The listing builds one solid part. Answer for the finished solid, in the listing's coordinates (mm). A direction names the side the tool comes from. Coordinates: 2 decimals unless noted, no trailing zeros. Write each loop counter-clockwise with the first axis right and the second up, starting at its lowest first coordinate (ties: lowest second). Pieces come first, ordered by that corner, then holes.
(1) Straight lines are drawn through the part: line 1 (Y direction, x = -12.5, z = 2.5); line 2 (X direction, y = 163, z = 4); line 3 (Y direction, x = -48.5, z = -1.5). For each, find the intervals that lie inside material, in ascending order.
(2) For a pull along Y with two mould halves and no side action, classify faces 6 (the flat face through (68, 129, 4.762)), 7 (the flat face through (-24, 197, 0)), 8 (the flat face through (-80, 197, 4.762)) as +Y half, -Y half, draft (parallel to the pull), parting line (faces both ways), or undercut.
(3) Which of the six approach directions +Z, -Z, +X, -X, +Y, -Y give full straight-line access (tool end or side, diameter ignored) to faces 1 (the flat face through (0, 118, 4.762)), 2 (the flat face through (68, 265, 4.762)), 3 (the flat face through (-69, 129, 4.762)), 4 (the flat face through (0, 276, 4.762)), 5 (the flat face through (-69, 265, 4.762))?
(4) The part is cut by section B-B on y = 95. Determine the outline of the cut face in (x, z).
(5) The part is cut by section A-A on x = 135.5. Determine the outline of the cut face in (y, z).
(6) The part is cut by section D-D on x = -44. Give the number of separate pieces and of enclosed holes in the cut face, plus the area to 3 significant figures.
(7) The part is cut by section C-C on z = -1.5. Determine the outline of the cut face in (x, y).
(8) Given P1, Ø9.5, axis at x = -86.5, y = 189, coming from the +Z side; P2, Ø3, axis at y = 130, z = 1, coming from the -X side; P3, Ø3, axis at x = -133.5, y = 176, coming from the -Z side; P4, Ø8, axis at x = 139.5, y = 163.5, coming from the +Z side, each flat-ended and moving along its own axis, determine where each tip first touches the part or whether it passes through.
from build123d import *
from OCP.BRepFilletAPI import BRepFilletAPI_MakeChamfer

# Parameters (mm, degrees)
SKETCH1_W           = 31.75
SKETCH1_H           = 38.1
SKETCH1_H_2         = 6.35
SKETCH1_W_2         = 6.35
SKETCH1_H_3         = 31.75
SKETCH1_W_3         = 38.1
BOSS_EXTRUDE1_DEPTH = 4.7625
SKETCH1_4_W         = 6.35
SKETCH1_4_H         = 31.75
SKETCH1_4_W_2       = 38.1
SKETCH1_4_W_3       = 31.75
SKETCH1_4_H_2       = 6.35
SKETCH1_4_H_3       = 38.1
BOSS_EXTRUDE2_DEPTH = 3.175
SKETCH1_5_W         = 38.1
SKETCH1_5_H         = 6.35
SKETCH1_5_W_2       = 63.5
SKETCH1_5_W_3       = 6.35
SKETCH1_5_H_2       = 38.1
SKETCH1_5_W_4       = 19.05
SKETCH1_5_H_3       = 139.7
SKETCH1_5_H_4       = 19.05
SKETCH1_5_H_5       = 158.75
SKETCH1_5_H_6       = 31.75
SKETCH1_5_W_5       = 31.75
BOSS_EXTRUDE3_DEPTH = 6.35
CHAMFER1_SIZE       = 25.4
CHAMFER1_SIZE2      = 3.175
CHAMFER2_SIZE       = 3.175
CHAMFER2_SIZE2      = 25.4
CHAMFER3_SIZE       = 38.1
CHAMFER3_SIZE2      = 3.175


with BuildPart() as part:
    # Sketch1 → Boss-Extrude1 (new body)
    with BuildSketch(Plane.XY):
        Polygon((-63.5, 171.45), (-95.25, 171.45), (-95.25, 101.6), (-25.4, 101.6), (-25.4, 133.35), (-63.5, 133.35), align=None)
        with Locations((-79.375, 196.85)):
            Rectangle(SKETCH1_W, SKETCH1_H)
        with Locations((-79.375, 174.625)):
            Rectangle(SKETCH1_W, SKETCH1_H_2)
        with Locations((-79.375, 219.075)):
            Rectangle(SKETCH1_W, SKETCH1_H_2)
        Polygon((-25.4, 260.35), (-25.4, 292.1), (-95.25, 292.1), (-95.25, 222.25), (-63.5, 222.25), (-63.5, 260.35), align=None)
        with Locations((-22.225, 276.225)):
            Rectangle(SKETCH1_W_2, SKETCH1_H_3)
        with Locations((0, 276.225)):
            Rectangle(SKETCH1_W_3, SKETCH1_H_3)
        with Locations((22.225, 276.225)):
            Rectangle(SKETCH1_W_2, SKETCH1_H_3)
        Polygon((95.25, 292.1), (25.4, 292.1), (25.4, 260.35), (63.5, 260.35), (63.5, 222.25), (95.25, 222.25), align=None)
        with Locations((79.375, 219.075)):
            Rectangle(SKETCH1_W, SKETCH1_H_2)
        with Locations((79.375, 196.85)):
            Rectangle(SKETCH1_W, SKETCH1_H)
        with Locations((79.375, 174.625)):
            Rectangle(SKETCH1_W, SKETCH1_H_2)
        Polygon((95.25, 101.6), (95.25, 171.45), (63.5, 171.45), (63.5, 133.35), (25.4, 133.35), (25.4, 101.6), align=None)
        with Locations((22.225, 117.475)):
            Rectangle(SKETCH1_W_2, SKETCH1_H_3)
        with Locations((0, 117.475)):
            Rectangle(SKETCH1_W_3, SKETCH1_H_3)
        with Locations((-22.225, 117.475)):
            Rectangle(SKETCH1_W_2, SKETCH1_H_3)
    extrude(amount=BOSS_EXTRUDE1_DEPTH)

    # Sketch1<4> → Boss-Extrude2 (add)
    with BuildSketch(Plane.XY):
        Polygon((95.25, 292.1), (25.4, 292.1), (25.4, 260.35), (63.5, 260.35), (63.5, 222.25), (95.25, 222.25), align=None)
        with Locations((22.225, 276.225)):
            Rectangle(SKETCH1_4_W, SKETCH1_4_H)
        with Locations((0, 276.225)):
            Rectangle(SKETCH1_4_W_2, SKETCH1_4_H)
        with Locations((-22.225, 276.225)):
            Rectangle(SKETCH1_4_W, SKETCH1_4_H)
        Polygon((-25.4, 260.35), (-25.4, 292.1), (-95.25, 292.1), (-95.25, 222.25), (-63.5, 222.25), (-63.5, 260.35), align=None)
        with Locations((-79.375, 219.075)):
            Rectangle(SKETCH1_4_W_3, SKETCH1_4_H_2)
        with Locations((-79.375, 196.85)):
            Rectangle(SKETCH1_4_W_3, SKETCH1_4_H_3)
        with Locations((-79.375, 174.625)):
            Rectangle(SKETCH1_4_W_3, SKETCH1_4_H_2)
        Polygon((-63.5, 171.45), (-95.25, 171.45), (-95.25, 101.6), (-25.4, 101.6), (-25.4, 133.35), (-63.5, 133.35), align=None)
        with Locations((-22.225, 117.475)):
            Rectangle(SKETCH1_4_W, SKETCH1_4_H)
        with Locations((0, 117.475)):
            Rectangle(SKETCH1_4_W_2, SKETCH1_4_H)
        Polygon((95.25, 101.6), (95.25, 171.45), (63.5, 171.45), (63.5, 133.35), (25.4, 133.35), (25.4, 101.6), align=None)
        with Locations((22.225, 117.475)):
            Rectangle(SKETCH1_4_W, SKETCH1_4_H)
        with Locations((79.375, 174.625)):
            Rectangle(SKETCH1_4_W_3, SKETCH1_4_H_2)
        with Locations((79.375, 196.85)):
            Rectangle(SKETCH1_4_W_3, SKETCH1_4_H_3)
        with Locations((79.375, 219.075)):
            Rectangle(SKETCH1_4_W_3, SKETCH1_4_H_2)
    extrude(amount=-BOSS_EXTRUDE2_DEPTH)

    # Sketch1<5> → Boss-Extrude3 (add)
    with BuildSketch(Plane.XY):
        with Locations((44.45, 219.075)):
            Rectangle(SKETCH1_5_W, SKETCH1_5_H)
        with Locations((127, 219.075)):
            Rectangle(SKETCH1_5_W_2, SKETCH1_5_H)
        with Locations((22.225, 219.075)):
            Rectangle(SKETCH1_5_W_3, SKETCH1_5_H)
        with Locations((0, 219.075)):
            Rectangle(SKETCH1_5_W, SKETCH1_5_H)
        with Locations((-22.225, 219.075)):
            Rectangle(SKETCH1_5_W_3, SKETCH1_5_H)
        with Locations((-44.45, 219.075)):
            Rectangle(SKETCH1_5_W, SKETCH1_5_H)
        with Locations((-22.225, 241.3)):
            Rectangle(SKETCH1_5_W_3, SKETCH1_5_H_2)
        with Locations((22.225, 241.3)):
            Rectangle(SKETCH1_5_W_3, SKETCH1_5_H_2)
        with Locations((22.225, 196.85)):
            Rectangle(SKETCH1_5_W_3, SKETCH1_5_H_2)
        with Locations((-22.225, 196.85)):
            Rectangle(SKETCH1_5_W_3, SKETCH1_5_H_2)
        with Locations((-22.225, 174.625)):
            Rectangle(SKETCH1_5_W_3, SKETCH1_5_H)
        with Locations((0, 174.625)):
            Rectangle(SKETCH1_5_W, SKETCH1_5_H)
        with Locations((22.225, 174.625)):
            Rectangle(SKETCH1_5_W_3, SKETCH1_5_H)
        with Locations((44.45, 174.625)):
            Rectangle(SKETCH1_5_W, SKETCH1_5_H)
        with Locations((22.225, 152.4)):
            Rectangle(SKETCH1_5_W_3, SKETCH1_5_H_2)
        with Locations((-22.225, 152.4)):
            Rectangle(SKETCH1_5_W_3, SKETCH1_5_H_2)
        with Locations((-44.45, 174.625)):
            Rectangle(SKETCH1_5_W, SKETCH1_5_H)
        with Locations((-127, 219.075)):
            Rectangle(SKETCH1_5_W_2, SKETCH1_5_H)
        with Locations((-127, 174.625)):
            Rectangle(SKETCH1_5_W_2, SKETCH1_5_H)
        with Locations((-168.275, 174.625)):
            Rectangle(SKETCH1_5_W_4, SKETCH1_5_H)
        with Locations((-168.275, 219.075)):
            Rectangle(SKETCH1_5_W_4, SKETCH1_5_H)
        with Locations((-22.225, 361.95)):
            Rectangle(SKETCH1_5_W_3, SKETCH1_5_H_3)
        with Locations((22.225, 361.95)):
            Rectangle(SKETCH1_5_W_3, SKETCH1_5_H_3)
        with Locations((22.225, 441.325)):
            Rectangle(SKETCH1_5_W_3, SKETCH1_5_H_4)
        with Locations((-22.225, 441.325)):
            Rectangle(SKETCH1_5_W_3, SKETCH1_5_H_4)
        with Locations((127, 174.625)):
            Rectangle(SKETCH1_5_W_2, SKETCH1_5_H)
        with Locations((168.275, 219.075)):
            Rectangle(SKETCH1_5_W_4, SKETCH1_5_H)
        with Locations((168.275, 174.625)):
            Rectangle(SKETCH1_5_W_4, SKETCH1_5_H)
        with Locations((22.225, 22.225)):
            Rectangle(SKETCH1_5_W_3, SKETCH1_5_H_5)
        with Locations((-22.225, 22.225)):
            Rectangle(SKETCH1_5_W_3, SKETCH1_5_H_5)
        with Locations((-22.225, 117.475)):
            Rectangle(SKETCH1_5_W_3, SKETCH1_5_H_6)
        with Locations((22.225, 117.475)):
            Rectangle(SKETCH1_5_W_3, SKETCH1_5_H_6)
        with Locations((-79.375, 174.625)):
            Rectangle(SKETCH1_5_W_5, SKETCH1_5_H)
        with Locations((-79.375, 219.075)):
            Rectangle(SKETCH1_5_W_5, SKETCH1_5_H)
        with Locations((-22.225, 276.225)):
            Rectangle(SKETCH1_5_W_3, SKETCH1_5_H_6)
        with Locations((22.225, 276.225)):
            Rectangle(SKETCH1_5_W_3, SKETCH1_5_H_6)
        with Locations((79.375, 219.075)):
            Rectangle(SKETCH1_5_W_5, SKETCH1_5_H)
        with Locations((79.375, 174.625)):
            Rectangle(SKETCH1_5_W_5, SKETCH1_5_H)
    extrude(amount=BOSS_EXTRUDE3_DEPTH)

    # Chamfer1: one chamfer whose edges measure the first distance from different faces: ONE call of the kernel's chamfer builder (chamfer() names one face for all edges)
    chamfer1_edges_1 = [part.edges().sort_by_distance(p)[0] for p in [
        (22.225, 450.85, 0),
    ]]
    chamfer1_side_1 = [part.faces().sort_by_distance(p)[0] for p in [
        (22.225, 371.475, 0),
    ]]
    chamfer1_edges_2 = [part.edges().sort_by_distance(p)[0] for p in [
        (-22.225, 450.85, 0),
    ]]
    chamfer1_side_2 = [part.faces().sort_by_distance(p)[0] for p in [
        (-22.225, 371.475, 0),
    ]]
    chamfer1_edges_3 = [part.edges().sort_by_distance(p)[0] for p in [
        (-177.8, 219.075, 0),
    ]]
    chamfer1_side_3 = [part.faces().sort_by_distance(p)[0] for p in [
        (-136.525, 219.075, 0),
    ]]
    chamfer1_edges_4 = [part.edges().sort_by_distance(p)[0] for p in [
        (-177.8, 174.625, 0),
    ]]
    chamfer1_side_4 = [part.faces().sort_by_distance(p)[0] for p in [
        (-136.525, 174.625, 0),
    ]]
    chamfer1 = BRepFilletAPI_MakeChamfer(part.part.solid().wrapped)
    for e in chamfer1_edges_1:
        chamfer1.Add(CHAMFER1_SIZE, CHAMFER1_SIZE2, e.wrapped, chamfer1_side_1[0].wrapped)  # the first distance lies on this face
    for e in chamfer1_edges_2:
        chamfer1.Add(CHAMFER1_SIZE, CHAMFER1_SIZE2, e.wrapped, chamfer1_side_2[0].wrapped)  # the first distance lies on this face
    for e in chamfer1_edges_3:
        chamfer1.Add(CHAMFER1_SIZE, CHAMFER1_SIZE2, e.wrapped, chamfer1_side_3[0].wrapped)  # the first distance lies on this face
    for e in chamfer1_edges_4:
        chamfer1.Add(CHAMFER1_SIZE, CHAMFER1_SIZE2, e.wrapped, chamfer1_side_4[0].wrapped)  # the first distance lies on this face
    add(Compound.cast(chamfer1.Shape()), mode=Mode.REPLACE)

    # Chamfer2: one chamfer whose edges measure the first distance from different faces: ONE call of the kernel's chamfer builder (chamfer() names one face for all edges)
    chamfer2_edges_1 = [part.edges().sort_by_distance(p)[0] for p in [
        (177.8, 219.075, 0),
    ]]
    chamfer2_side_1 = [part.faces().sort_by_distance(p)[0] for p in [
        (177.8, 219.075, 3.175),
    ]]
    chamfer2_edges_2 = [part.edges().sort_by_distance(p)[0] for p in [
        (177.8, 174.625, 0),
    ]]
    chamfer2_side_2 = [part.faces().sort_by_distance(p)[0] for p in [
        (177.8, 174.625, 3.175),
    ]]
    chamfer2 = BRepFilletAPI_MakeChamfer(part.part.solid().wrapped)
    for e in chamfer2_edges_1:
        chamfer2.Add(CHAMFER2_SIZE, CHAMFER2_SIZE2, e.wrapped, chamfer2_side_1[0].wrapped)  # the first distance lies on this face
    for e in chamfer2_edges_2:
        chamfer2.Add(CHAMFER2_SIZE, CHAMFER2_SIZE2, e.wrapped, chamfer2_side_2[0].wrapped)  # the first distance lies on this face
    add(Compound.cast(chamfer2.Shape()), mode=Mode.REPLACE)

    # Chamfer3: one chamfer whose edges measure the first distance from different faces: ONE call of the kernel's chamfer builder (chamfer() names one face for all edges)
    chamfer3_edges_1 = [part.edges().sort_by_distance(p)[0] for p in [
        (-22.225, -57.15, 0),
    ]]
    chamfer3_side_1 = [part.faces().sort_by_distance(p)[0] for p in [
        (-22.225, 22.225, 0),
    ]]
    chamfer3_edges_2 = [part.edges().sort_by_distance(p)[0] for p in [
        (22.225, -57.15, 0),
    ]]
    chamfer3_side_2 = [part.faces().sort_by_distance(p)[0] for p in [
        (22.225, 22.225, 0),
    ]]
    chamfer3 = BRepFilletAPI_MakeChamfer(part.part.solid().wrapped)
    for e in chamfer3_edges_1:
        chamfer3.Add(CHAMFER3_SIZE, CHAMFER3_SIZE2, e.wrapped, chamfer3_side_1[0].wrapped)  # the first distance lies on this face
    for e in chamfer3_edges_2:
        chamfer3.Add(CHAMFER3_SIZE, CHAMFER3_SIZE2, e.wrapped, chamfer3_side_2[0].wrapped)  # the first distance lies on this face
    add(Compound.cast(chamfer3.Shape()), mode=Mode.REPLACE)


solid = part.part
Model answer:
1. line 1: y = 101.6 to 133.35, 171.45 to 177.8, 215.9 to 222.25, 260.35 to 292.1
1. line 2: x = -95.25 to -63.5, -25.4 to -19.05, 19.05 to 25.4, 63.5 to 95.25
1. line 3: y = 101.6 to 133.35, 260.35 to 292.1
2. face 6: draft
2. face 7: undercut
2. face 8: undercut
3. face 1: +Z, -Y
3. face 2: +Z, +X, +Y
3. face 3: +Z, -X, -Y
3. face 4: +Z, +Y
3. face 5: +Z, -X, +Y
4. outline: (-25.4, 0) - (-19.05, 0) - (-19.05, 6.35) - (-25.4, 6.35) - close; (19.05, 0) - (25.4, 0) - (25.4, 6.35) - (19.05, 6.35) - close
5. outline: (171.45, 0) - (177.8, 0) - (177.8, 6.35) - (171.45, 6.35) - close; (215.9, 0) - (222.25, 0) - (222.25, 6.35) - (215.9, 6.35) - close
6. separate pieces: 4
6. enclosed holes: 0
6. area: 585 mm2
7. outline: (-95.25, 101.6) - (95.25, 101.6) - (95.25, 292.1) - (-95.25, 292.1) - close; hole (-63.5, 133.35) - (63.5, 133.35) - (63.5, 260.35) - (-63.5, 260.35) - close
8. P1: stops at z = 4.76
8. P2: stops at x = -95.25
8. P3: stops at z = 0
8. P4: passes through
